Here's how the part is built. I have some questions about the finished solid (model axes, mm). Give positions to 0.01 mm unless a question says otherwise; leave off trailing zeros. Loops run counter-clockwise (first coordinate to the right, second up) from the corner with the lowest first, then second, coordinate; pieces in that order, holes last.
Q1. Will these pins go through, and if not, where does the flat tip stop? P1, Ø18.5, axis at x = 200, y = 373.5, coming from the +Z side; P2, Ø2.5, axis at y = 394, z = 1.5, coming from the -X side; P3, Ø2.5, axis at y = 393, z = 2.5, coming from the +X side.
Q2. If we section it at A-A (x = 200): Please give me the cut outline in (y, z).
Q3. We'd pull the mould along X, two halves only. Please class faces 1 (the face through (190.874, 366.502, 2.535)), 2 (the face through (197, 201, 5)): +X half, -X half, draft (parallel to the pull), parting line (faces both ways), or undercut.
Q4. I need wall thicknesses on line 1 (X direction, y = 358, z = 3); line 2 (X direction, y = 389, z = 3.5); line 3 (Y direction, x = 215.5, z = 1.5). Which ranges of each line are inside material? Lowest first, please.
Q5. If we section it at B-B (z = 2.1): Give the number of separate pieces and of enclosed holes in the cut face, plus the area to 3 significant figures.
from build123d import *

# Parameters (mm, degrees)
SKETCH1_W           = 400
SKETCH1_H           = 397
BOSS_EXTRUDE1_DEPTH = 5
SKETCH2_R           = 1.55
CUT_EXTRUDE1_DEPTH  = 6
SKETCH3_R           = 11.5
CUT_EXTRUDE2_DEPTH  = 6
SKETCH4_W           = 157
SKETCH4_H           = 10
CUT_EXTRUDE3_DEPTH  = 6
SKETCH5_R           = 4
CUT_EXTRUDE4_DEPTH  = 5


with BuildPart() as part:
    # Sketch1 → Boss-Extrude1 (new body)
    with BuildSketch(Plane.XY):
        with Locations((200, 198.5)):
            Rectangle(SKETCH1_W, SKETCH1_H)
    extrude(amount=BOSS_EXTRUDE1_DEPTH)

    # Sketch2 → Cut-Extrude1 (cut, through all)
    with BuildSketch(Plane.XY.offset(5)):
        with Locations((215.5, 389)):
            Circle(SKETCH2_R)
        with Locations((215.5, 358)):
            Circle(SKETCH2_R)
        with Locations((184.5, 358)):
            Circle(SKETCH2_R)
        with Locations((184.5, 389)):
            Circle(SKETCH2_R)
    extrude(amount=-CUT_EXTRUDE1_DEPTH, mode=Mode.SUBTRACT)

    # Sketch3 → Cut-Extrude2 (cut, through all)
    with BuildSketch(Plane.XY.offset(5)):
        with Locations((200, 373.5)):
            Circle(SKETCH3_R)
    extrude(amount=-CUT_EXTRUDE2_DEPTH, mode=Mode.SUBTRACT)

    # Sketch4 → Cut-Extrude3 (cut, through all)
    with BuildSketch(Plane.XY.offset(5)):
        with Locations((321.5, 392)):
            Rectangle(SKETCH4_W, SKETCH4_H)
        with Locations((78.5, 392)):
            Rectangle(SKETCH4_W, SKETCH4_H)
    extrude(amount=-CUT_EXTRUDE3_DEPTH, mode=Mode.SUBTRACT)

    # Sketch5 → Cut-Extrude4 (cut)
    with BuildSketch(Plane.XY.offset(5)):
        with Locations((25, 367.03)):
            Circle(SKETCH5_R)
        with Locations((25, 20.03)):
            Circle(SKETCH5_R)
        with Locations((375, 20.03)):
            Circle(SKETCH5_R)
        with Locations((375, 367.03)):
            Circle(SKETCH5_R)
    extrude(amount=-CUT_EXTRUDE4_DEPTH, mode=Mode.SUBTRACT)


solid = part.part
Check sheet entries:
1. P1: passes through
1. P2: stops at x = 157
1. P3: stops at x = 243
2. outline: (0, 0) - (362, 0) - (362, 5) - (0, 5) - close; (385, 0) - (397, 0) - (397, 5) - (385, 5) - close
3. face 1: undercut
3. face 2: draft
4. line 1: x = 0 to 182.95, 186.05 to 213.95, 217.05 to 400
4. line 2: x = 157 to 182.95, 186.05 to 213.95, 217.05 to 243
4. line 3: y = 0 to 356.45, 359.55 to 387.45, 390.55 to 397
5. separate pieces: 1
5. enclosed holes: 9
5. area: 155,000 mm2
